Autodesk Inventor part; units mm, degrees
ref_plane "YZ Plane" through (0, 0, 0) normal (1, 0, 0) x (0, 1, 0)
ref_plane "XZ Plane" through (0, 0, 0) normal (0, 1, 0) x (-1, 0, 0)
ref_plane "XY Plane" through (0, 0, 0) normal (0, 0, 1) x (1, 0, 0)
sketch "Sketch1" plane through (0, 0, 0) normal (0, 0, 1) x (1, 0, 0)
  line L0 (-109.7639, -7) -> (-109.7639, 7)
  line L1 (-105.2639, 5) -> (-90.2639, 5) construction
  line L2 (-90.2639, 5) -> (-90.2639, -5) construction
  line L3 (-90.2639, -5) -> (-105.2639, -5) construction
  line L4 (-105.2639, -5) -> (-105.2639, 5) construction
  line L5 (-105.2639, 5) -> (-90.2639, -5) construction
  line L6 (-90.2639, 5) -> (-105.2639, -5) construction
  circle A0 centre (-105.2639, 5) radius 1.6
  circle A1 centre (-90.2639, 5) radius 1.6
  circle A2 centre (-105.2639, -5) radius 1.6
  circle A3 centre (-90.2639, -5) radius 1.6
  circle A4 centre (90.7361, 45) radius 1.6
  circle A5 centre (105.7361, 45) radius 1.6
  circle A6 centre (90.7361, 35) radius 1.6
  circle A7 centre (105.7361, 35) radius 1.6
  line L7 (-109.7639, 7) -> (-106.7639, 10)
  line L8 (-109.7639, -7) -> (-106.7639, -10)
  line L9 (87.2361, 50) -> (107.2361, 50)
  line L10 (110.2361, 47) -> (110.2361, -7)
  line L11 (107.2361, -10) -> (87.1625, -10)
  circle A8 centre (105.7361, -5) radius 1.6
  circle A9 centre (105.7361, 5) radius 1.6
  circle A10 centre (90.7361, -5) radius 1.6
  circle A11 centre (90.7361, 5) radius 1.6
  line L12 (90.7361, 45) -> (105.7361, 45) construction
  line L13 (105.7361, 35) -> (105.7361, 5) construction
  line L14 (107.2361, 50) -> (110.2361, 47)
  line L15 (110.2361, -7) -> (107.2361, -10)
  line L16 (87.2361, 50) -> (66.2361, 10)
  line L17 (87.1625, -10) -> (66, -10)
  line L18 (-106.7639, 10) -> (66.2361, 10)
  line L19 (66, -10) -> (-106.7639, -10)
  point P0 (0, 0)
  point P1 (0.2361, 0)
  point P2 (98.4723, 19.4096)
  point P3 (-97.7639, 0)
  point P4 (0.2361, 0)
  point P5 (98.2361, 45)
  point P6 (105.7361, 20)
  point P7 (98.2361, 20)
  dimension "d4" = 15
  dimension "d5" = 10
  dimension "d6" = 12
  dimension "d8" = 3.2
  dimension "d20" = 15
  dimension "d21" = 10
  dimension "d22" = 15
  dimension "d23" = 10
  dimension "d24" = 30
  dimension "d31" = 4.5
  dimension "d32" = 5
  dimension "d34" = 220
  dimension "d35" = 3
  dimension "d36" = 3
  dimension "d37" = 3
  dimension "d38" = 3
  dimension "d39" = 20
extrude "Extrusion1" add sketch "Sketch1" along normal blind 10
sketch "Sketch3" plane through (0, 0, 10) normal (0, 0, 1) x (1, 0, 0)
  point P0 (0, 0)
properties part number "HorizontalBridge"
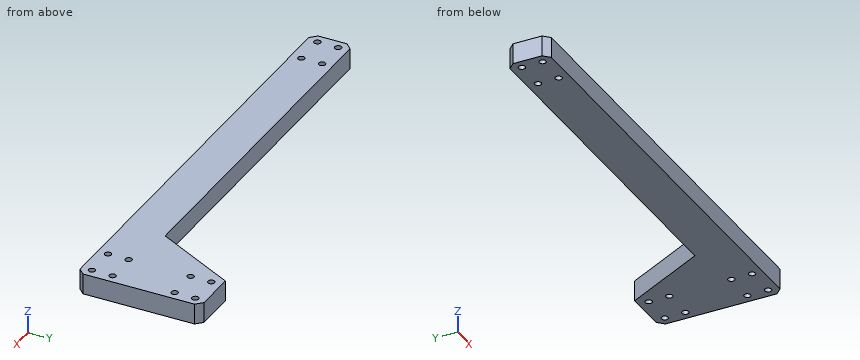
Model file for the job. Use its own axes, mm. Round coordinates to 2 decimals unless told otherwise and drop trailing zeros. Write each loop counter-clockwise with the first axis right and the second up, starting at its lowest first coordinate (ties: lowest second). Pieces come first, ordered by that corner, then holes. Notation, with made-up numbers: (51, 80.5) - (104, 80.5) arc R22 ccw to (104, 91.5) - close; hole circle Ø10 at (34, -39.75). An arc over 180 degrees is marked (long way). One line per item, written item: value.
(1) Cut at C-C, the plane y = 30.5. Give the cut face in (x, z), plus the area to 3 significant figures.
Values follow:
outline: (77, 0) - (110.24, 0) - (110.24, 10) - (77, 10) - close
area: 332 mm²
(2) Wall check: probe 1 along Y at (x, z) = (-23.5, 2.25); probe 2 along Y at (x, z) = (68, 7.25); probe 3 along X at (y, z) = (37.5, 9). Give the ranges that are in metal, low to high.
Values follow:
probe 1: y = -10 to 10
probe 2: y = -10 to 13.36
probe 3: x = 80.67 to 110.24
(3) Cut at B-B, the plane x = -59. Give the cut face in (y, z), plus the area to 3 significant figures.
Values follow:
outline: (-10, 0) - (10, 0) - (10, 10) - (-10, 10) - close
area: 200 mm²
(4) Drop flat-ended pins along their axis: P1, Ø5, axis at y = 10, z = 2, coming from the -X side; P2, Ø5, axis at x = 17.5, z = 3.5, coming from the +Y side; P3, Ø3.5, axis at x = 105.74, y = -5, coming from the -Z side. Give the stop position or say it passes through.
Values follow:
P1: stops at x = -109.26
P2: stops at y = 10
P3: stops at z = 0
(5) Cut at A-A, the plane z = 3.5. Give the number of separate pieces and of enclosed holes in the cut face, plus the area to 3 significant figures.
Values follow:
separate pieces: 1
enclosed holes: 12
area: 5,630 mm²
